Can you work these out from the model? Positions are in its coordinate system, mm. A direction names the side the tool comes from. Round coordinates to 2 decimals unless told otherwise and drop trailing zeros. Write each loop counter-clockwise with the first axis right and the second up, starting at its lowest first coordinate (ties: lowest second). Pieces come first, ordered by that corner, then holes. Notation, with made-up numbers: (-24.75, -7.75) - (10.25, -7.75) arc R20 ccw to (10.25, 25.25) - close; hole circle Ø3 at (17, 3.5). An arc over 180 degrees is marked (long way). One line per item, written item: value. Start each with the question number.
(1) On a 3-axis mill with a long thin cutter (end or side, diameter ignored), from which of +Z, -Z, +X, -X, +Y, -Y can I reach the whole of each face in a straight line? I mean faces 5 (the face through (25, 23, 25)), 6 (the face through (0, -24, 49)). Say none if no direction works.
(2) Thinking about a two-plate mould opening in X: for faces 1 (the face through (25, -23, 25)), 2 (the face through (-2.17, -9.76, 25.82)), 3 (the face through (-24, 0, 49)), 4 (the face through (0, -25, 25)), which applies, +X half, -X half, draft (parallel to the pull), parting line (faces both ways), or undercut?
(3) If I drill on L1, parallel to Y at x = 0, z = 28.5; L2, parallel to Y at x = -6, z = 24.5; L3, parallel to X at y = 9, z = 32, over which ranges is the centre line in solid material (lowest first)? Write a range as from..to.
(4) I want a section at A-A on x = 0. List the corners of the cut face in (y, z) for me, plus the area to 3 significant figures.
(5) I'm going to push flat-ended pins straight in: pin 1 Ø12.5 at (y, z) = (-14.5, 19) entering from +X; pin 2 Ø4 at (x, y) = (36.5, -8.5) entering from -Z; pin 3 Ø12 at (y, z) = (-12, 21.5) entering from +X. Where does each tip first touch, or does it pass through?
(6) I want a section at B-B on x = 24. List the corners of the cut face in (y, z) for me.
from build123d import *

# Parameters (mm, degrees)
F0_W     = 50
F0_H     = 50
F1_DEPTH = 50
F2_R     = 10
F3_DEPTH = 50.001
F4_SIZE  = 2
F5_R     = 3


with BuildPart() as f1:
    # F0 (on Top) → F1 (new body)
    with BuildSketch(Plane.XY):
        Rectangle(F0_W, F0_H)
    extrude(amount=F1_DEPTH)

    # F2 (on face) → F3 (cut, through all)
    with BuildSketch(Plane.XY.offset(50)):
        Circle(F2_R)
    extrude(amount=-F3_DEPTH, mode=Mode.SUBTRACT)

    # F4
    f4_edges = [f1.edges().sort_by_distance(p)[0] for p in [
        (0, -25, 50),
        (-25, 0, 50),
        (25, 0, 50),
        (0, 25, 50),
        (-10, 0, 50),
    ]]
    chamfer(f4_edges, length=F4_SIZE)

    # F5
    f5_edges = [f1.edges().sort_by_distance(p)[0] for p in [
        (0, -25, 0),
        (-25, 0, 0),
        (25, 0, 0),
        (0, 25, 0),
        (-10, 0, 0),
    ]]
    fillet(f5_edges, radius=F5_R)

    # F6 (on Front) → F7 (revolve)
    with BuildSketch(Plane.XZ):
        with BuildLine():
            Line((45, 25.5), (25, 25.5))
            Line((25, 25.5), (25, 3))
            add(Edge.make_bspline(
                [(45, 25.5), (44.5258021355, 20.7176618278), (42.3149203915, 12.2219088735), (31.248183921, 3.7772532087), (25, 3)],
                knots=[0, 0, 0, 0, 0.4587105615, 1, 1, 1, 1], degree=3))
        make_face()
    revolve(axis=Axis((35, 0, 25.5), (1, 0, 0)))


solid = f1.part
Established:
1. face 5: +X, +Y
1. face 6: +Z, +X, -X, -Y
2. face 1: +X half
2. face 2: undercut
2. face 3: -X half
2. face 4: draft
3. L1: -25..-10, 10..25
3. L2: -25..-8, 8..25
3. L3: -25..-4.36, 4.36..41.63
4. outline: (-25, 3) arc R3 ccw to (-22, 0) - (-13, 0) arc R3 ccw to (-10, 3) - (-10, 48) - (-12, 50) - (-23, 50) - (-25, 48) - close; (10, 3) arc R3 ccw to (13, 0) - (22, 0) arc R3 ccw to (25, 3) - (25, 48) - (23, 50) - (12, 50) - (10, 48) - close
4. area: 1,480 mm2
5. pin 1: x = 42.46
5. pin 2: z = 8.76
5. pin 3: x = 43.71
6. outline: (-25, 3) arc R3 ccw to (-24, 0.76) - (24, 0.76) arc R3 ccw to (25, 3) - (25, 48) - (24, 49) - (-24, 49) - (-25, 48) - close
